Input: part model. Units: mm. Frame: model coordinates. Give positions to 0.01 mm unless a question says otherwise; leave off trailing zeros. Write each loop counter-clockwise with the first axis right and the second up, starting at its lowest first coordinate (ties: lowest second). Pieces come first, ordered by that corner, then holes. Notation, with made-up numbers: (-29, -39.75) - (-16, -39.75) arc R35 ccw to (-16, -3.75) - close; hole circle Ø6 at (-20, 56.5). An arc over 180 degrees is marked (long way). Use a Markdown table: item, result. Add a question column.
1. Section query B-B, the plane z = -265. Return loops of the section in (x, y).
2. Section query A-A, the plane x = 0. Return loops of the section in (y, z), plus the area to 3 significant figures.
3. Pin query (flat end, axial travel): pin 1 (3 mm diameter, centred on x = 3, y = 1.5, fed in from -Z); pin 2 (2 mm diameter, centred on y = -1.5, z = -224, fed in from +X); pin 3 (1 mm diameter, centred on x = 3, y = 3.5, fed in from -Z); pin 4 (2 mm diameter, centred on x = 1, z = -145.5, fed in from +Y). Return the tip coordinate at first contact, or that it passes through.
4. Material intervals for probe 1 along Y at (x, z) = (0, -10); probe 2 along Z at (x, y) = (-1.5, -3.75); probe 3 along Z at (x, y) = (0, -2.5), sorted ascending.
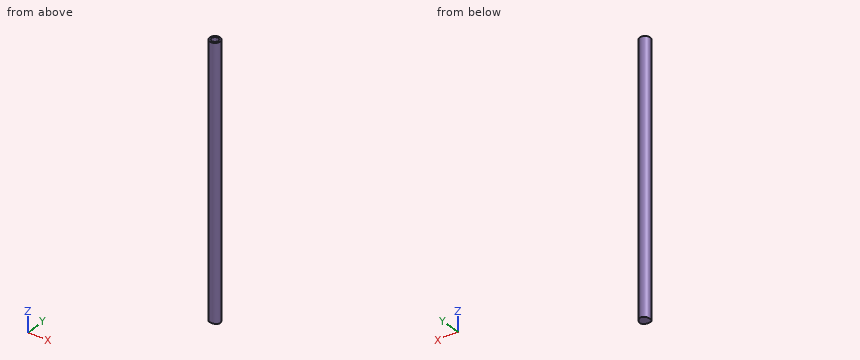
Autodesk Inventor part; units mm, degrees
ref_plane "YZ Plane" through (0, 0, 0) normal (1, 0, 0) x (0, 1, 0)
ref_plane "XZ Plane" through (0, 0, 0) normal (0, 1, 0) x (-1, 0, 0)
ref_plane "XY Plane" through (0, 0, 0) normal (0, 0, 1) x (1, 0, 0)
sketch "Sketch1" plane through (0, 0, 0) normal (0, 1, 0) x (-1, 0, 0)
  line L0 (0, -456) -> (0, 76) construction
  line L1 (-1.27, 0) -> (7.62, 0) construction
  line L2 (0, 0) -> (6.35, 0)
  line L3 (6.35, 0) -> (6.35, -350)
  line L4 (6.35, -350) -> (0, -350)
  line L5 (0, -350) -> (0, 0)
  dimension "d0" = 350
  dimension "d1" = 6.35
revolve "Revolution1" add sketch "Sketch1" angle 360 about axis through (0, 0, -350) along (0, 0, 1)
sketch "Sketch2" plane through (0, 0, 0) normal (0, 1, 0) x (-1, 0, 0)
  line L0 (6.35, -350) -> (-6.35, -350)
  circle A0 centre (0, -350) radius 20
  point P0 (0, 0)
  dimension "d3" = 40
extrude "Extrusion1" cut sketch "Sketch2" along normal through all both and the other way through all
sketch "Sketch3" plane through (0, 0, 0) normal (0, 0, 1) x (1, 0, 0)
  circle A0 centre (0, 0) radius 4.2164
  point P0 (0, 0)
  dimension "d6" = 8.4328
extrude "Extrusion2" cut sketch "Sketch3" against normal blind 50.8
thread "Thread1"
properties part number "Suspenion_Arm_Assembly_V2_Member"
Result sheet:
| question | item | result |
|---|---|---|
| 1 | outline | circle Ø12.7 at (0, 0) |
| 2 | outline | (-6.35, -330) - (6.35, -330) - (6.35, 0) - (4.22, 0) - (4.22, -50.8) - (-4.22, -50.8) - (-4.22, 0) - (-6.35, 0) - close |
| 2 | area | 3,760 mm² |
| 3 | pin 1 | stops at z = -330.51 |
| 3 | pin 2 | stops at x = 6.33 |
| 3 | pin 3 | stops at z = -330.31 |
| 3 | pin 4 | stops at y = 6.35 |
| 4 | probe 1 | y = -6.35 to -4.22, 4.22 to 6.35 |
| 4 | probe 2 | z = -330.06 to -50.8 |
| 4 | probe 3 | z = -330 to -50.8 |
